Verification items for the finished model (mm, model axes). A direction names the side the tool comes from. Give positions to 0.01 mm unless a question says otherwise; leave off trailing zeros. Loops run counter-clockwise (first coordinate to the right, second up) from the corner with the lowest first, then second, coordinate; pieces in that order, holes last. Notation, with made-up numbers: M 42.5,21.5 L 56.5,21.5 A20 cw 56.5,25.5 Z; hole C 61.5,-2.75 d1. An arc over 180 degrees is marked long. Write each question's results on one line, items separated by ' | '. Start each with the question number.
```python
from build123d import *

# Parameters (mm, degrees)
F1_DEPTH = 5
F3_DEPTH = 25


with BuildPart() as f1:
    # F0 (on Front) → F1 (new body)
    with BuildSketch(Plane.XZ):
        with BuildLine():
            ThreePointArc((0, 5), (1.464466, 1.464466), (5, 0))
            Line((5, 0), (6, 0))
            ThreePointArc((6, 0), (15.395129, 3.306774), (20.647917, 11.769127))
            ThreePointArc((20.647917, 11.769127), (17.754785, 15.176301), (21, 18.25))
            Line((21, 18.25), (21, 25))
            ThreePointArc((21, 25), (22.464466, 28.535534), (26, 30))
            Line((26, 30), (474, 30))
            ThreePointArc((474, 30), (477.535534, 28.535534), (479, 25))
            Line((479, 25), (479, 18.25))
            ThreePointArc((479, 18.25), (482.245215, 15.176301), (479.352083, 11.769127))
            ThreePointArc((479.352083, 11.769127), (484.604871, 3.306774), (494, 0))
            Line((494, 0), (495, 0))
            ThreePointArc((495, 0), (498.535534, 1.464466), (500, 5))
            Line((500, 5), (500, 55))
            Line((500, 55), (485, 55))
            ThreePointArc((485, 55), (475, 45), (465, 55))
            Line((465, 55), (455, 55))
            ThreePointArc((455, 55), (445, 45), (435, 55))
            Line((435, 55), (425, 55))
            ThreePointArc((425, 55), (415, 45), (405, 55))
            Line((405, 55), (395, 55))
            ThreePointArc((395, 55), (385, 45), (375, 55))
            Line((375, 55), (365, 55))
            ThreePointArc((365, 55), (355, 45), (345, 55))
            Line((345, 55), (335, 55))
            ThreePointArc((335, 55), (325, 45), (315, 55))
            Line((315, 55), (305, 55))
            ThreePointArc((305, 55), (295, 45), (285, 55))
            Line((285, 55), (275, 55))
            ThreePointArc((275, 55), (265, 45), (255, 55))
            Line((255, 55), (245, 55))
            ThreePointArc((245, 55), (235, 45), (225, 55))
            Line((225, 55), (215, 55))
            ThreePointArc((215, 55), (205, 45), (195, 55))
            Line((195, 55), (185, 55))
            ThreePointArc((185, 55), (175, 45), (165, 55))
            Line((165, 55), (155, 55))
            ThreePointArc((155, 55), (145, 45), (135, 55))
            Line((135, 55), (125, 55))
            ThreePointArc((125, 55), (115, 45), (105, 55))
            Line((105, 55), (95, 55))
            ThreePointArc((95, 55), (85, 45), (75, 55))
            Line((75, 55), (65, 55))
            ThreePointArc((65, 55), (55, 45), (45, 55))
            Line((45, 55), (35, 55))
            ThreePointArc((35, 55), (25, 45), (15, 55))
            Line((15, 55), (0, 55))
            Line((0, 55), (0, 5))
        make_face()
    extrude(amount=F1_DEPTH)

    # F2 (on face) → F3 (join)
    with BuildSketch(Plane(origin=(0, 0, 0), x_dir=(-1, 0, 0), z_dir=(0, 1, 0))):
        with BuildLine():
            ThreePointArc((-500, 5), (-498.535534, 1.464466), (-495, 0))
            Line((-495, 0), (-494, 0))
            ThreePointArc((-494, 0), (-484.604871, 3.306774), (-479.352083, 11.769127))
            ThreePointArc((-479.352083, 11.769127), (-482.245215, 15.176301), (-479, 18.25))
            Line((-479, 18.25), (-479, 25))
            ThreePointArc((-479, 25), (-477.535534, 28.535534), (-474, 30))
            Line((-474, 30), (-26, 30))
            ThreePointArc((-26, 30), (-22.464466, 28.535534), (-21, 25))
            Line((-21, 25), (-21, 18.25))
            ThreePointArc((-21, 18.25), (-17.754785, 15.176301), (-20.647917, 11.769127))
            ThreePointArc((-20.647917, 11.769127), (-15.395129, 3.306774), (-6, 0))
            Line((-6, 0), (-5, 0))
            ThreePointArc((-5, 0), (-1.464466, 1.464466), (0, 5))
            Line((0, 5), (0, 55))
            Line((0, 55), (-15, 55))
            ThreePointArc((-15, 55), (-25, 45), (-35, 55))
            Line((-35, 55), (-45, 55))
            ThreePointArc((-45, 55), (-55, 45), (-65, 55))
            Line((-65, 55), (-75, 55))
            ThreePointArc((-75, 55), (-85, 45), (-95, 55))
            Line((-95, 55), (-105, 55))
            ThreePointArc((-105, 55), (-115, 45), (-125, 55))
            Line((-125, 55), (-135, 55))
            ThreePointArc((-135, 55), (-145, 45), (-155, 55))
            Line((-155, 55), (-165, 55))
            ThreePointArc((-165, 55), (-175, 45), (-185, 55))
            Line((-185, 55), (-195, 55))
            ThreePointArc((-195, 55), (-205, 45), (-215, 55))
            Line((-215, 55), (-225, 55))
            ThreePointArc((-225, 55), (-235, 45), (-245, 55))
            Line((-245, 55), (-255, 55))
            ThreePointArc((-255, 55), (-265, 45), (-275, 55))
            Line((-275, 55), (-285, 55))
            ThreePointArc((-285, 55), (-295, 45), (-305, 55))
            Line((-305, 55), (-315, 55))
            ThreePointArc((-315, 55), (-325, 45), (-335, 55))
            Line((-335, 55), (-345, 55))
            ThreePointArc((-345, 55), (-355, 45), (-365, 55))
            Line((-365, 55), (-375, 55))
            ThreePointArc((-375, 55), (-385, 45), (-395, 55))
            Line((-395, 55), (-405, 55))
            ThreePointArc((-405, 55), (-415, 45), (-425, 55))
            Line((-425, 55), (-435, 55))
            ThreePointArc((-435, 55), (-445, 45), (-455, 55))
            Line((-455, 55), (-465, 55))
            ThreePointArc((-465, 55), (-475, 45), (-485, 55))
            Line((-485, 55), (-500, 55))
            Line((-500, 55), (-500, 5))
        make_face()
        with BuildLine():
            Line((-343.16784, 52.999999), (-336.83216, 52.999999))
            ThreePointArc((-336.83216, 52.999999), (-325, 42.999999), (-313.16784, 52.999999))
            Line((-313.16784, 52.999999), (-306.83216, 52.999999))
            ThreePointArc((-306.83216, 52.999999), (-295, 42.999999), (-283.16784, 52.999999))
            Line((-283.16784, 52.999999), (-276.83216, 52.999999))
            ThreePointArc((-276.83216, 52.999999), (-265, 42.999999), (-253.16784, 52.999999))
            Line((-253.16784, 52.999999), (-246.83216, 52.999999))
            ThreePointArc((-246.83216, 52.999999), (-235, 42.999999), (-223.16784, 52.999999))
            Line((-223.16784, 52.999999), (-216.83216, 52.999999))
            ThreePointArc((-216.83216, 52.999999), (-205, 42.999999), (-193.16784, 52.999999))
            Line((-193.16784, 52.999999), (-186.83216, 52.999999))
            ThreePointArc((-186.83216, 52.999999), (-175, 42.999999), (-163.16784, 52.999999))
            Line((-163.16784, 52.999999), (-156.83216, 52.999999))
            ThreePointArc((-156.83216, 52.999999), (-145, 42.999999), (-133.16784, 52.999999))
            Line((-133.16784, 52.999999), (-126.83216, 52.999999))
            ThreePointArc((-126.83216, 52.999999), (-115, 42.999999), (-103.16784, 52.999999))
            Line((-103.16784, 52.999999), (-96.83216, 52.999999))
            ThreePointArc((-96.83216, 52.999999), (-85, 42.999999), (-73.16784, 52.999999))
            Line((-73.16784, 52.999999), (-66.83216, 52.999999))
            ThreePointArc((-66.83216, 52.999999), (-55, 42.999999), (-43.16784, 52.999999))
            Line((-43.16784, 52.999999), (-36.83216, 52.999999))
            ThreePointArc((-36.83216, 52.999999), (-25, 42.999999), (-13.16784, 52.999999))
            Line((-13.16784, 52.999999), (-2.000001, 52.999999))
            Line((-2.000001, 52.999999), (-2.000001, 5))
            ThreePointArc((-2.000001, 5), (-2.87868, 2.87868), (-5, 2.000001))
            Line((-5, 2.000001), (-6, 2.000001))
            ThreePointArc((-6, 2.000001), (-13.454792, 4.349833), (-18.214583, 10.549836))
            ThreePointArc((-18.214583, 10.549836), (-15.768605, 15.441606), (-18.999999, 19.854122))
            Line((-18.999999, 19.854122), (-18.999999, 25))
            ThreePointArc((-18.999999, 25), (-21.050252, 29.949748), (-26, 32.000001))
            Line((-26, 32.000001), (-474, 32.000001))
            ThreePointArc((-474, 32.000001), (-478.949748, 29.949748), (-481.000001, 25))
            Line((-481.000001, 25), (-481.000001, 19.854122))
            ThreePointArc((-481.000001, 19.854122), (-484.231395, 15.441606), (-481.785417, 10.549836))
            ThreePointArc((-481.785417, 10.549836), (-486.545208, 4.349833), (-494, 2.000001))
            Line((-494, 2.000001), (-495, 2.000001))
            ThreePointArc((-495, 2.000001), (-497.12132, 2.87868), (-497.999999, 5))
            Line((-497.999999, 5), (-497.999999, 52.999999))
            Line((-497.999999, 52.999999), (-486.83216, 52.999999))
            ThreePointArc((-486.83216, 52.999999), (-475, 42.999999), (-463.16784, 52.999999))
            Line((-463.16784, 52.999999), (-456.83216, 52.999999))
            ThreePointArc((-456.83216, 52.999999), (-445, 42.999999), (-433.16784, 52.999999))
            Line((-433.16784, 52.999999), (-426.83216, 52.999999))
            ThreePointArc((-426.83216, 52.999999), (-415, 42.999999), (-403.16784, 52.999999))
            Line((-403.16784, 52.999999), (-396.83216, 52.999999))
            ThreePointArc((-396.83216, 52.999999), (-385, 42.999999), (-373.16784, 52.999999))
            Line((-373.16784, 52.999999), (-366.83216, 52.999999))
            ThreePointArc((-366.83216, 52.999999), (-355, 42.999999), (-343.16784, 52.999999))
        make_face(mode=Mode.SUBTRACT)
    extrude(amount=F3_DEPTH)


solid = f1.part
```
1. Section check A-A, the plane x = 85. Record the boundary of the cut face in (y, z).
2. Set-up check for faces 3 (the face through (485, 10, 3)), 4 (the face through (484.224, 12.325, 15.522)), 5 (the face through (115, 10, 45)): record each of +Z, -Z, +X, -X, +Y, -Y from which the full face is reachable in a straight line by a thin tool's end or side.
3. Depth check by flat-ended pin: pin 1 Ø1.5 at (x, y) = (207, 11.5) entering from +Z; pin 2 Ø3 at (x, y) = (310.5, 10.5) entering from -Z; pin 3 Ø12.5 at (x, y) = (236.5, 14.5) entering from +Z. Enter the tip coordinate at first touch or a pass-through.
4. Release check for a two-part mould opening along X. For faces 1 (the face through (340, 10, 55)), 2 (the face through (55, 10, 45)) record: released by +X, released by -X, zero draft, split by the parting line, or undercut.
5. Thickness scan on probe 1 along X at (y, z) = (15.25, 34); probe 2 along Z at (x, y) = (339.5, 19); probe 3 along X at (y, z) = (7, 13). Record the ranges inside material, lowest first.
6. Section check B-B, the plane x = 327. Record the boundary of the cut face in (y, z).
Filled sheet:
1) outline: M -5,30 L 25,30 L 25,32 L 0,32 L 0,43 L 25,43 L 25,45 L -5,45 Z
2) face 3: -Z, +Y, -Y | face 4: +Y | face 5: +Z, +Y, -Y
3) pin 1: z = 45.39 | pin 2: z = 30 | pin 3: z = 48.68
4) face 1: zero draft | face 2: undercut
5) probe 1: 0 to 2, 498 to 500 | probe 2: 30 to 32, 53 to 55 | probe 3: 0 to 2, 16.15 to 18.44, 481.56 to 483.85, 498 to 500
6) outline: M -5,30 L 25,30 L 25,32 L 0,32 L 0,43.17 L 25,43.17 L 25,45.2 L -5,45.2 Z
